```python
from build123d import *

# Parameters (mm, degrees)
F0_R     = 10
F1_DEPTH = 5
F2_R     = 5
F3_DEPTH = 85
F4_R     = 2


with BuildPart() as f1:
    # F0 (on Top) → F1 (new body)
    with BuildSketch(Plane.XY):
        Circle(F0_R)
    extrude(amount=F1_DEPTH)

    # F2 (on face) → F3 (join)
    with BuildSketch(Plane.XY.offset(5)):
        Circle(F2_R)
    extrude(amount=F3_DEPTH)

    # F4
    f4_edges = [f1.edges().sort_by_distance(p)[0] for p in [
        (-5, 0, 90),
        (-10, 0, 0),
    ]]
    fillet(f4_edges, radius=F4_R)


solid = f1.part
```
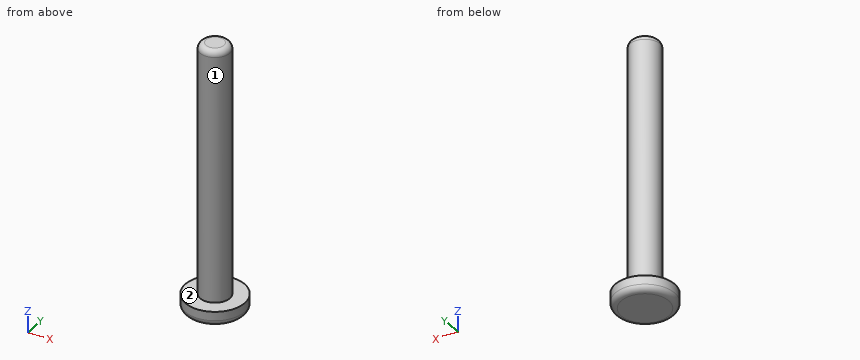
CAD build for the part. Positions are in the model's coordinates, mm. Face numbers are marked on the shaded views. Round coordinates to 2 decimals unless told otherwise and drop trailing zeros. Order: outer loops, then holes, each group sorted by start corner. A loop starts at its lowest first (then second) coordinate and runs counter-clockwise, first axis right, second up. Notation, with made-up numbers: (-37, 70.25) - (-22, 70.25) arc R13 cw to (-22, 82.25) - close; hole circle Ø10 at (58, -0.5). An arc over 180 degrees is marked (long way). Answer in a Markdown table with one row per item. Add a question column.
(1) Band-saw the part on A-A on x = 0. List the corners of the cut face in (y, z), and give its area (3 significant figures).
(2) Mould opens along Y. For the marked faces 1 and 2 say: +Y half, -Y half, draft (parallel to the pull), parting line (faces both ways), or undercut.
(3) Drop flat-ended pins along their axis: pin 1 Ø6 at (x, y) = (-7.5, 5) entering from +Z; pin 2 Ø5 at (y, z) = (1, 17.5) entering from -X; pin 3 Ø3 at (y, z) = (-5.5, 17.5) entering from -X. Give the stop position or say it passes through.
(4) Band-saw the part on B-B on z = 70. List the corners of the cut face in (x, y), and give its area (3 significant figures).
(5) Probe L1, parallel to Z at x = 0.25, y = -3.25; L2, parallel to Z at x = -0.25, y = -6.25; L3, parallel to X at y = 4.25, z = 51. List the from-to ranges inside material, lowest first. Write a range as [from, to].
Data:
| question | item | result |
|---|---|---|
| 1 | outline | (-10, 2) arc R2 ccw to (-8, 0) - (8, 0) arc R2 ccw to (10, 2) - (10, 5) - (5, 5) - (5, 88) arc R2 ccw to (3, 90) - (-3, 90) arc R2 ccw to (-5, 88) - (-5, 5) - (-10, 5) - close |
| 1 | area | 947 mm^2 |
| 2 | face 1 | parting line |
| 2 | face 2 | draft |
| 3 | pin 1 | stops at z = 5 |
| 3 | pin 2 | stops at x = -5 |
| 3 | pin 3 | stops at x = -3 |
| 4 | outline | circle Ø10 at (0, 0) |
| 4 | area | 78.5 mm^2 |
| 5 | L1 | z = [0, 89.98] |
| 5 | L2 | z = [0, 5] |
| 5 | L3 | x = [-2.63, 2.63] |
